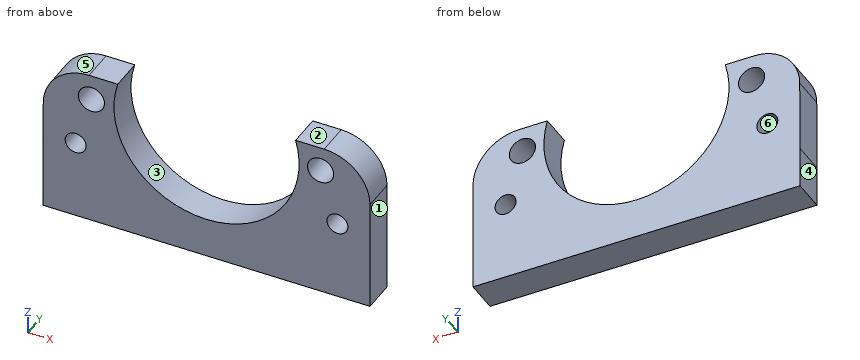
```python
from build123d import *

# Parameters (mm, degrees)
PAD018_DEPTH    = 5
FILLET_R        = 7
SKETCH045_R     = 2
SKETCH045_R_2   = 1.6
POCKET014_DEPTH = 5


with BuildPart() as part:
    # Sketch044 → Pad018 (new body)
    with BuildSketch(Plane.XZ):
        with BuildLine():
            ThreePointArc((-13.565707, 79.497418), (-0.091594, 61.343037), (13.616485, 79.321409))
            Line((24.977643, 79.321409), (13.616485, 79.321409))
            Line((24.977643, 61.321409), (24.977643, 79.321409))
            Line((24.977643, 61.321409), (24.977643, 55.203457))
            Line((24.977643, 55.203457), (-24.990618, 55.203457))
            Line((-24.990618, 55.203457), (-24.990618, 61.497418))
            Line((-24.926865, 79.497418), (-24.990618, 61.497418))
            Line((-24.926865, 79.497418), (-13.565707, 79.497418))
        make_face()
    extrude(amount=-PAD018_DEPTH)

    # Fillet
    fillet_edges = [part.edges().sort_by_distance(p)[0] for p in [
        (24.977643, 2.5, 79.321409),
        (-24.926865, 2.5, 79.497418),
    ]]
    fillet(fillet_edges, radius=FILLET_R)

    # Sketch045 (on Face5 of Fillet) → Pocket014 (cut)
    with BuildSketch(Plane(origin=(0, 5, 0), x_dir=(1, 0, 0), z_dir=(0, 1, 0))):
        with Locations((-17.590132, -75.56945)):
            Circle(SKETCH045_R)
        with Locations((17.428322, -75.561134)):
            Circle(SKETCH045_R)
        with Locations((-20.002373, -67.402222)):
            Circle(SKETCH045_R_2)
        with Locations((20.00708, -67.407166)):
            Circle(SKETCH045_R_2)
    extrude(amount=-POCKET014_DEPTH, mode=Mode.SUBTRACT)


with BuildPart() as part_1:
    # Body020 placement: moved
    add(part.part.moved(Location((0, 13, 0))))


solid = part_1.part
```
Work out the finished part from the listing and answer in its coordinate system (mm). Face numbers are marked on the shaded views. A direction names the side the tool comes from. Coordinates: 2 decimals unless noted, no trailing zeros. Write each loop counter-clockwise with the first axis right and the second up, starting at its lowest first coordinate (ties: lowest second). Pieces come first, ordered by that corner, then holes. Notation, with made-up numbers: (13, -8.75) - (29, -8.75) arc R12 ccw to (29, 11.25) - close; hole circle Ø11 at (34.5, 74.25). An arc over 180 degrees is marked (long way). Answer as a JSON object with one key per item and string values.
Q1. Find section A-A (z = 70.75). Write down the section's boundary in (x, y).
Results list:
{"outline": "(-24.96, 13) - (-13.33, 13) - (-13.33, 18) - (-24.96, 18) - close; (13.33, 13) - (24.98, 13) - (24.98, 18) - (13.33, 18) - close"}
Q2. Find section B-B (y = 14.2). Write down the section's boundary in (x, z), plus the area to 3 significant figures.
Results list:
{"outline": "(-24.99, 55.2) - (24.98, 55.2) - (24.98, 72.32) arc R7 ccw to (17.98, 79.32) - (13.62, 79.32) arc R14.15 cw (long way) to (-13.57, 79.5) - (-17.95, 79.5) arc R7 ccw to (-24.95, 72.52) - (-24.99, 61.5) - close; hole circle Ø3.2 at (-20, 67.4); hole circle Ø4 at (-17.59, 75.57); hole circle Ø4 at (17.43, 75.56); hole circle Ø3.2 at (20.01, 67.41)", "area": "723 mm^2"}
Q3. Which of the six approach directions +Z, -Z, +X, -X, +Y, -Y give full straight-line access (tool end or side, diameter ignored) to the marked faces 1 and 2?
Results list:
{"face 1": "+Z, -Z, +X, +Y, -Y", "face 2": "+Z, +X, +Y, -Y"}
Q4. Find section C-C (z = 77). Write down the section's boundary in (x, y).
Results list:
{"outline": "(-23.31, 13) - (-18.99, 13) - (-18.99, 18) - (-23.31, 18) - close; (-16.19, 13) - (-14.06, 13) - (-14.06, 18) - (-16.19, 18) - close; (14.06, 13) - (16.04, 13) - (16.04, 18) - (14.06, 18) - close; (18.82, 13) - (23.18, 13) - (23.18, 18) - (18.82, 18) - close"}
Q5. Consider L1, parallel to X at y = 15.1, z = 68.75; L2, parallel to X at y = 16.5, z = 67.25; L3, parallel to Z at x = 17.5, y = 15.35. Determine where each line is inside the solid, lowest interval first. Write a range as from..to.
Results list:
{"L1": "x = -24.96..-20.86, -19.14..-12.44, 12.44..19.14, 20.88..24.98", "L2": "x = -24.97..-21.6, -18.41..-11.5, 11.5..18.41, 21.6..24.98", "L3": "z = 55.2..73.56, 77.56..79.32"}
Q6. For a pull along Z with two mould halves and no side action, classify the marked faces 3, 4, 5 and 6 as pulls with the +Z half, pulls with the -Z half, needs draft (parallel to the pull), parting line crosses it, or undercut.
Results list:
{"face 3": "undercut", "face 4": "needs draft", "face 5": "pulls with the +Z half", "face 6": "undercut"}
Q7. Find section D-D (x = 0). Write down the section's boundary in (y, z), plus the area to 3 significant figures.
Results list:
{"outline": "(13, 55.2) - (18, 55.2) - (18, 61.34) - (13, 61.34) - close", "area": "30.7 mm^2"}
